Autodesk Inventor part; units mm, degrees
ref_plane "Work Plane1" through (1.525, 0, 0) normal (0, 0, 1) x (1, 0, 0)
ref_plane "YZ Plane" through (0, 0, 0) normal (1, 0, 0) x (0, 1, 0)
ref_plane "XZ Plane" through (0, 0, 0) normal (0, 1, 0) x (-1, 0, 0)
sketch "Sketch1" plane through (0, 0, 0) normal (0, 0, 1) x (1, 0, 0)
  line L0 (0, 4) -> (30, 4)
  line L1 (30, 4) -> (30, 0)
  line L2 (30, 0) -> (0, 0)
  line L3 (-6, 0) -> (36, 0)
  line L4 (0, -0.8) -> (0, 4.8)
  line L5 (0, 4) -> (0, 0)
  dimension "d2" = 8
  dimension "d59" = 30
revolve "Body" add sketch "Sketch1" angle 360 about axis through (30, 0, 0) along (-1, 0, 0)
sketch "Sketch2" plane through (0, 0, 0) normal (-1, 0, 0) x (0, 0, 1)
  line L0 (0, 7.5056) -> (6.5, 3.7528)
  line L1 (6.5, 3.7528) -> (6.5, -3.7528)
  line L2 (6.5, -3.7528) -> (0, -7.5056)
  line L3 (0, -7.5056) -> (-6.5, -3.7528)
  line L4 (-6.5, -3.7528) -> (-6.5, 3.7528)
  line L5 (-6.5, 3.7528) -> (0, 7.5056)
  line L6 (-9.1, 0) -> (9.1, 0)
  line L7 (0, 10.5078) -> (0, -10.5078)
  point P0 (0, 0)
  point P1 (0, 0)
  dimension "d11" = 13
extrude "Head" add sketch "Sketch2" along normal blind 5.68
sketch "Sketch4" plane through (0, 0, 0) normal (0, 0, 1) x (1, 0, 0)
  line L0 (-4.9294, 7.8) -> (-5.68, 6.5)
  line L1 (-1.1, 0) -> (-0.234, 0)
  line L2 (-6.7692, 0) -> (0.8552, 0)
  line L3 (-5.68, 7.8) -> (-4.9294, 7.8)
  line L4 (-5.68, 6.5) -> (-5.68, 7.8)
  line L5 (0, 9.36) -> (0, -1.56)
  dimension "d65" = 13
  dimension "d67" = 30
  dimension "d68" = 15.6
  dimension "d69" = 5.68
revolve "Chamfer1" cut sketch "Sketch4" angle 360 about axis through (-1.1, 0, 0) along (1, 0, 0)
thread "Thread"
chamfer "Chamfer2" distance 0.7668 distance2 0.7669 1 edges at (30, -4, 0) measured on face at (30, -0.998, 0.8842)
fillet "Fillet" radius 0.1 1 edges at (0, -4, 0)
ref_plane "Work Plane1" through (1.525, 0, 0) normal (0, 0, 1) x (1, 0, 0)
equation "\"d2\" = GD"
equation "\"d59\" = NLG"
equation "\"d11\" = SW"
equation "\"d3\" = KOH"
equation "\"d15\" = GEL"
equation "\"d6\" = -0.5 * SPD + 0.5 * GD"
equation "\"d71\" = RR"
equation "\"d65\" = SW"
equation "\"d67\" = ANG1"
equation "\"d68\" = 1.2 * SW"
equation "\"d69\" = KOH"
equation "\"NLG\" = 30"
equation "\"GD\" = NND"
equation "\"BDM\" = NND"
equation "\"KOH\" = 5.68"
equation "\"GEL\" = 22"
equation "\"SW\" = 13"
equation "\"SW0\" = SW"
equation "\"SPD\" = NND - 1.2269 * PTC"
equation "\"SD2\" = NND"
equation "\"SD\" = 0"
equation "\"ANG1\" = 30deg"
equation "\"GAL\" = 0.61345 * PTC"
equation "\"GUL\" = 0.61345 * PTC"
equation "\"RR\" = 0.1"
equation "\"RR1\" = 0.4"
equation "\"GD1\" = THREADDIA - 1.2269 * PTC"
equation "\"THREADDIA\" = 8"
equation "\"TOA\" = 30deg"
equation "\"PTC\" = 1.25"
equation "\"KOH1\" = 3.7"
equation "\"NND\" = 8"
equation "\"E0\" = 1.155 * SW"
properties part number "ANSI B18.2.3.5M - M8 x 1.25 x 30" material "Steel, Mild"
CAD build for the part. Positions are in the model's coordinates, mm. A direction names the side the tool comes from. Give positions to 0.01 mm unless a question says otherwise; leave off trailing zeros. Order: outer loops, then holes, each group sorted by start corner. A loop starts at its lowest first (then second) coordinate and runs counter-clockwise, first axis right, second up. Notation, with made-up numbers: M 36.5,28.5 L 67.5,28.5 A26 ccw 67.5,54.5 Z; hole C 76,36.25 d7. An arc over 180 degrees is marked long. Put each result on its own line as item: value. Start each with the question number.
(1) Which spindle directions (+Z, -Z, +X, -X, +Y, -Y) get a long thin tool onto all of the face, cutting with end or side? Do faces 1 (the flat face through (-2.8, -5.66, -3.2)), 2 (the cylindrical face through (14.87, -0.867, -3.905)). Say none if no direction does.
(2) Drill centre lines: line 1 along X through (y, z) = (-5.25, 3.5); line 2 along Y through (x, z) = (23.5, -2.5); line 3 along Z through (x, y) = (13.5, 2.25). Where is each one in solid material? Low to high.
(3) Flat gauge pins, fed straight in: pin 1 Ø3 at (x, y) = (11.5, -4) entering from -Z; pin 2 Ø1.5 at (x, y) = (17, 3) entering from -Z; pin 3 Ø3 at (x, y) = (21, 3) entering from +Z. Where does each tip first touch, or does it go through?
(4) Saw through at A-A, the plane x = -1.5. Write the cut outline in (y, z), then the cut area to 3 significant figures.
Check result:
1. face 1: -Z, +X, -X, -Y
1. face 2: +X
2. line 1: x = -5.68 to 0
2. line 2: y = -3.12 to 3.12
2. line 3: z = -3.31 to 3.31
3. pin 1: stops at z = -3.12
3. pin 2: stops at z = -3.31
3. pin 3: stops at z = 3.71
4. outline: M -7.51,0 L -3.75,-6.5 L 3.75,-6.5 L 7.51,0 L 3.75,6.5 L -3.75,6.5 Z
4. area: 146 mm2
